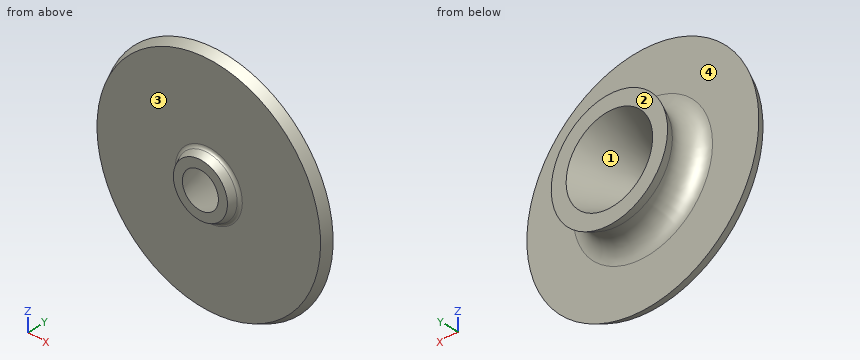
from build123d import *

# Parameters (mm, degrees)
FILLET2_R = 12.7
FILLET3_R = 2.54


with BuildPart() as part:
    # Sketch1 → Revolve2 (revolve)
    with BuildSketch(Plane.XY, mode=Mode.PRIVATE) as revolve2_sk:
        Polygon((-12.7, -0.571707157), (-30.466321776, 37.528292843), (-40.975996454, 37.528292843), (-29.131781937, 12.128292843), (-50.190671319, 12.128292843), (-81.680155327, 12.128292843), (-78.719101698, 5.778292843), (-22.011053629, 5.778292843), (-19.05, -0.571707157), align=None)
    revolve(revolve2_sk.sketch.rotate(Axis((0, 0, 0), (0, 1, 0)), 270), axis=Axis((0, 0, 0), (0, 1, 0)))

    # Fillet2
    fillet2_edges = [part.edges().sort_by_distance(p)[0] for p in [
        (0, 12.128292843, 29.131781937),
    ]]
    fillet(fillet2_edges, radius=FILLET2_R)

    # Fillet3
    fillet3_edges = [part.edges().sort_by_distance(p)[0] for p in [
        (0, 5.778292843, 22.011053629),
    ]]
    fillet(fillet3_edges, radius=FILLET3_R)


solid = part.part
Build history of the part. All positions in model axes, mm. Face numbers are marked on the shaded views. A direction names the side the tool comes from. Round coordinates to 2 decimals unless told otherwise and drop trailing zeros. Write each loop counter-clockwise with the first axis right and the second up, starting at its lowest first coordinate (ties: lowest second). Pieces come first, ordered by that corner, then holes. Notation, with made-up numbers: M 66.25,-19 L 75.25,-19 A22 cw 75.25,10 Z; hole C 7,61.25 d10. An arc over 180 degrees is marked long. Answer in a Markdown table with one row per item.
1. Saw through at B-B (z = 0). List the corners of the cut face in (x, y), and give its area (3 significant figures).
Geometry check:
| item | result |
|---|---|
| outline | M -81.68,12.13 L -78.72,5.78 L -23.63,5.78 A2.54 cw -21.33,4.31 L -19.05,-0.57 L -12.7,-0.57 L -30.47,37.53 L -40.98,37.53 L -37.56,30.2 A12.7 cw -49.07,12.13 Z; M 12.7,-0.57 L 19.05,-0.57 L 21.33,4.31 A2.54 cw 23.63,5.78 L 78.72,5.78 L 81.68,12.13 L 49.07,12.13 A12.7 cw 37.56,30.2 L 40.98,37.53 L 30.47,37.53 Z |
| area | 1,600 mm2 |
2. Saw through at D-D (y = 24). List the corners of the cut face in (x, z), and give its area (3 significant figures).
Geometry check:
| item | result |
|---|---|
| outline | C 0,0 d72.79; hole C 0,0 d48.32 |
| area | 2,330 mm2 |
3. Saw through at A-A (x = 0). List the corners of the cut face in (y, z).
Geometry check:
| item | result |
|---|---|
| outline | M -0.57,-19.05 L 4.31,-21.33 A2.54 cw 5.78,-23.63 L 5.78,-78.72 L 12.13,-81.68 L 12.13,-49.07 A12.7 cw 30.2,-37.56 L 37.53,-40.98 L 37.53,-30.47 L -0.57,-12.7 Z; M -0.57,12.7 L 37.53,30.47 L 37.53,40.98 L 30.2,37.56 A12.7 cw 12.13,49.07 L 12.13,81.68 L 5.78,78.72 L 5.78,23.63 A2.54 cw 4.31,21.33 L -0.57,19.05 Z |
4. Saw through at C-C (y = 8.5). List the corners of the cut face in (x, z).
Geometry check:
| item | result |
|---|---|
| outline | C 0,0 d159.98; hole C 0,0 d33.86 |
5. Mould opens along X. For the marked faces 1 and 2 say: +X half, -X half, draft (parallel to the pull), parting line (faces both ways), or undercut.
Geometry check:
| item | result |
|---|---|
| face 1 | undercut |
| face 2 | draft |
6. Which spindle directions (+Z, -Z, +X, -X, +Y, -Y) get a long thin tool onto all of the face, cutting with end or side? Do the marked faces 3 and 4. Say none if no direction does.
Geometry check:
| item | result |
|---|---|
| face 3 | -Y |
| face 4 | +Y |
7. Probe L1, parallel to Y at x = 31, z = -5.5; L2, parallel to Y at x = -43, z = -50.5; L3, parallel to X at y = 9.5, z = 12.5. List the from-to ranges inside material, lowest first. Write a range as [from, to].
Geometry check:
| item | result |
|---|---|
| L1 | [5.78, 37.53] |
| L2 | [5.78, 12.13] |
| L3 | [-79.48, -12.1], [12.1, 79.48] |
8. Flat gauge pins, fed straight in: P1, Ø2, axis at y = 28.5, z = -1, coming from the +X side; P2, Ø2, axis at x = -22.5, y = 17, coming from the +Z side; P3, Ø1, axis at y = 11.5, z = 44, coming from the +X side; P4, Ø2, axis at y = 3.5, z = 63.5, coming from the -X side. Where does each tip first touch, or does it go through?
Geometry check:
| item | result |
|---|---|
| P1 | x = 37.24 |
| P2 | z = 33.18 |
| P3 | x = 68.89 |
| P4 | through |
